Input: part model. Units: mm. Frame: model coordinates. A direction names the side the tool comes from. Give positions to 0.01 mm unless a question says otherwise; leave off trailing zeros. Loops run counter-clockwise (first coordinate to the right, second up) from the corner with the lowest first, then second, coordinate; pieces in that order, holes last.
from build123d import *

# Parameters (mm, degrees)
SKETCH1_R         = 1.143
MAINBODY_DEPTH    = 6.096
SKETCH2_OUTSIDE_W = 13.71
SKETCH2_OUTSIDE_H = 26.41
SKETCH2_OUTSIDE_R = 0.635
SIDETRIM_DEPTH    = 19.939


with BuildPart() as part:
    # Sketch1 → MainBody (new body)
    with BuildSketch(Plane(origin=(0, 0, 0), x_dir=(0, 0, -1), z_dir=(1, 0, 0))):
        with BuildLine():
            Line((0, 0), (0, 10.16))
            Line((0, 10.16), (3.048, 10.16))
            Line((3.048, 10.16), (3.048, 11.176))
            Line((3.048, 11.176), (18.787804319, 15.24))
            Line((18.787804319, 15.24), (18.864004319, 14.944878669))
            Line((18.864004319, 14.944878669), (3.3528, 10.939902935))
            Line((3.3528, 10.939902935), (3.3528, 10.16))
            Line((3.3528, 10.16), (6.0198, 10.16))
            Line((6.0198, 10.16), (6.0198, 10.6934))
            ThreePointArc((6.0198, 10.6934), (7.0104, 11.684), (8.001, 10.6934))
            Line((8.001, 10.6934), (8.001, 10.16))
            Line((8.001, 10.16), (9.779, 10.16))
            Line((9.779, 10.16), (10.287, 9.525))
            Line((10.287, 9.525), (19.939, 9.525))
            Line((19.939, 9.525), (19.939, 0))
            Line((19.939, 0), (18.415, 0))
            Line((18.415, 0), (18.415, -3.556))
            Line((18.415, -3.556), (17.907, -3.556))
            Line((17.907, -3.556), (17.907, 0))
            Line((17.907, 0), (11.049, 0))
            Line((11.049, 0), (11.049, -3.556))
            Line((11.049, -3.556), (10.541, -3.556))
            Line((10.541, -3.556), (10.541, 0))
            Line((10.541, 0), (2.413, 0))
            Line((2.413, 0), (2.413, -3.556))
            Line((2.413, -3.556), (1.905, -3.556))
            Line((1.905, -3.556), (1.905, 0))
            Line((1.905, 0), (0, 0))
        make_face()
        with Locations(Location((4.953, 2.286, 0), (0, 0, 180))):
            Circle(SKETCH1_R, mode=Mode.SUBTRACT)
        with Locations(Location((14.986, 2.286, 0), (0, 0, 180))):
            Circle(SKETCH1_R, mode=Mode.SUBTRACT)
    extrude(amount=MAINBODY_DEPTH)

    # Sketch2 outside → SideTrim (cut)
    # profile 1 of 2: a face of its own
    with BuildSketch(Plane.XY):
        with Locations((3.048, 5.842)):
            Rectangle(SKETCH2_OUTSIDE_W, SKETCH2_OUTSIDE_H)
        Polygon((0, 10.16), (1.0287, 10.16), (1.0287, 15.24), (5.0673, 15.24), (5.0673, 10.16), (6.096, 10.16), (6.096, 0), (4.6736, 0), (4.6736, -3.556), (1.4224, -3.556), (1.4224, 0), (0, 0), align=None, mode=Mode.SUBTRACT)
    # profile 2 of 2: a face of its own
    with BuildSketch(Plane.XY):
        with Locations(Location((3.048, -2.286, 0), (0, 0, 270))):
            Circle(SKETCH2_OUTSIDE_R)
    extrude(amount=-SIDETRIM_DEPTH, mode=Mode.SUBTRACT)


solid = part.part
(1) Cut plane A-A (y = -1.25). Return the cut outline in (x, z) (3 decimals), and give its area (3 significant figures).
Values follow:
outline: (1.422, -18.415) - (4.674, -18.415) - (4.674, -17.907) - (1.422, -17.907) - close; (1.422, -11.049) - (4.674, -11.049) - (4.674, -10.541) - (1.422, -10.541) - close; (1.422, -2.413) - (4.674, -2.413) - (4.674, -1.905) - (1.422, -1.905) - close
area: 4.95 mm2
(2) Cut plane D-D (z = -12). Return the cut outline in (x, y) (3 decimals).
Values follow:
outline: (0, 0) - (6.096, 0) - (6.096, 9.525) - (0, 9.525) - close; (1.029, 13.173) - (5.067, 13.173) - (5.067, 13.487) - (1.029, 13.487) - close
(3) Cut plane C-C (x = 2). Count the separate pieces of the cut face and the enclosed holes in it, and give its area (3 significant figures).
Values follow:
separate pieces: 1
enclosed holes: 2
area: 201 mm2
(4) Ray query, probe 1 along Z at (x, y) = (3.25, -1) (3 decimals); probe 2 along Z at (x, y) = (2.5, 10.5); probe 3 along Y at (x, z) = (4.25, -4). Return the intervals inside material, ascending.
Values follow:
probe 1: z = -18.415 to -17.907, -11.049 to -10.541, -2.413 to -1.905
probe 2: z = -8 to -6.02, -3.35 to -3.05
probe 3: y = 0 to 1.65, 2.92 to 10.16, 11.11 to 11.42
(5) Pin query (flat end, axial travel): pin 1 Ø2.5 at (y, z) = (13, -13) entering from +X; pin 2 Ø1 at (x, y) = (2.5, -2.5) entering from -Z (3 decimals); pin 3 Ø1 at (x, z) = (2, -9.5) entering from +Y; pin 4 Ø3.5 at (y, z) = (2.286, -14.986) entering from -X. Return the tip coordinate at first contact, or that it passes through.
Values follow:
pin 1: stops at x = 5.07
pin 2: stops at z = -18.415
pin 3: stops at y = 12.97
pin 4: stops at x = 0
(6) Mould query, pull axis Z, two halves, no side actions, for faces 1 (the flat face through (3, 0, -10)), 2 (the flat face through (0, 5, -10)), 3 (the flat face through (3.02, 13.18, -10.81)). Classes: +Z half, -Z half, draft (parallel to the pull), parting line (faces both ways), or undercut.
Values follow:
face 1: undercut
face 2: draft
face 3: +Z half
(7) Reachability of faces 4 (the flat face through (3, -1, -17.907)), 5 (the flat face through (3, 9.525, -15)), 6 (the flat face through (1.029, 11, -7)) from +Z, -Z, +X, -X, +Y, -Y: full face, straight path, thin tool, end or side. Return the list, or none.
Values follow:
face 4: +X, -X, -Y
face 5: -Z, +X, -X
face 6: +Z, -Z, -X, +Y
(8) Cut plane B-B (z = -4.25). Return the cut outline in (x, y), and give its area (3 significant figures).
Values follow:
outline: (0, 0) - (6.1, 0) - (6.1, 1.38) - (0, 1.38) - close; (0, 3.19) - (6.1, 3.19) - (6.1, 10.16) - (0, 10.16) - close; (1.03, 11.17) - (5.07, 11.17) - (5.07, 11.49) - (1.03, 11.49) - close
area: 52.2 mm2
